Work out the finished part from the listing and answer in its coordinate system (mm). Give positions to 0.01 mm unless a question says otherwise; leave off trailing zeros. Order: outer loops, then holes, each group sorted by start corner. A loop starts at its lowest first (then second) coordinate and runs counter-clockwise, first axis right, second up.
```python
from build123d import *

# Parameters (mm, degrees)
F0_W      = 505
F0_H      = 60
F1_DEPTH  = 10
F2_W      = 505
F2_H      = 2.3
F3_DEPTH  = 5.5
F4_W      = 505
F4_H      = 2.3
F5_DEPTH  = 2.5
F7_D      = 3.3
F7_DEPTH  = 13.5
F7_TIP    = 0.9914200214
F9_D      = 3.3
F9_DEPTH  = 15
F9_TIP    = 0.9914200214
F11_D     = 3.3
F11_DEPTH = 15
F11_TIP   = 0.9914200214


with BuildPart() as f1:
    # F0 (on Front) → F1 (new body)
    with BuildSketch(Plane.XZ):
        Rectangle(F0_W, F0_H)
    extrude(amount=F1_DEPTH)

    # F2 (on face) → F3 (cut)
    with BuildSketch(Plane.XZ.offset(10)):
        with Locations((0, -27.05)):
            Rectangle(F2_W, F2_H)
    extrude(amount=-F3_DEPTH, mode=Mode.SUBTRACT)

    # F4 (on face) → F5 (cut)
    with BuildSketch(Plane.XZ.offset(10)):
        with Locations((0, 4.15)):
            Rectangle(F4_W, F4_H)
    extrude(amount=-F5_DEPTH, mode=Mode.SUBTRACT)

    # F7
    with Locations(Plane.XY.offset(30)):
        with Locations((-210, -5), (-70, -5), (70, -5), (210, -5)):
            Hole(F7_D / 2, depth=F7_DEPTH)
            with Locations((0, 0, -(F7_DEPTH + F7_TIP / 2))):  # 118° drill point
                Cone(0, F7_D / 2, F7_TIP, mode=Mode.SUBTRACT)

    # F9
    with Locations(Plane(origin=(-252.5, 0, 0), x_dir=(0, -1, 0), z_dir=(-1, 0, 0))):
        with Locations((5, 24), (5, -15)):
            Hole(F9_D / 2, depth=F9_DEPTH)
            with Locations((0, 0, -(F9_DEPTH + F9_TIP / 2))):  # 118° drill point
                Cone(0, F9_D / 2, F9_TIP, mode=Mode.SUBTRACT)

    # F11
    with Locations(Plane.YZ.offset(252.5)):
        with Locations((-4.5, -15), (-4.5, 24)):
            Hole(F11_D / 2, depth=F11_DEPTH)
            with Locations((0, 0, -(F11_DEPTH + F11_TIP / 2))):  # 118° drill point
                Cone(0, F11_D / 2, F11_TIP, mode=Mode.SUBTRACT)


solid = f1.part
```
1. The part is cut by section A-A (x = -15). Write down the section's boundary in (y, z), then the cut area to 3 significant figures.
Findings below:
outline: (-10, -30) - (0, -30) - (0, 30) - (-10, 30) - (-10, 5.3) - (-7.5, 5.3) - (-7.5, 3) - (-10, 3) - (-10, -25.9) - (-4.5, -25.9) - (-4.5, -28.2) - (-10, -28.2) - close
area: 582 mm2
2. Straight lines are drawn through the part: probe 1 along Z at (x, y) = (-100, -8.75); probe 2 along X at (y, z) = (-5, 22.5); probe 3 along X at (y, z) = (-5, 21.75). For each, find the intervals that lie inside material, in ascending order.
Findings below:
probe 1: z = -30 to -28.2, -25.9 to 3, 5.3 to 30
probe 2: x = -237.41 to -211.65, -208.35 to -71.65, -68.35 to 68.35, 71.65 to 208.35, 211.65 to 237.46
probe 3: x = -252.5 to -211.65, -208.35 to -71.65, -68.35 to 68.35, 71.65 to 208.35, 211.65 to 252.5
3. Given P1, Ø3, axis at y = -4.5, z = 24, coming from the +X side; P2, Ø2, axis at y = -4.5, z = -15, coming from the -X side; P3, Ø2, axis at x = -210, y = -5, coming from the +Z side, each flat-ended and moving along its own axis, determine where each tip first touches the part or whether it passes through.
Findings below:
P1: stops at x = 237.41
P2: stops at x = -237.41
P3: stops at z = 16.11
